```python
from build123d import *

# Parameters (mm, degrees)
SKETCH1_W           = 5
SKETCH1_H           = 15
BOSS_EXTRUDE1_DEPTH = 7
CUT_EXTRUDE3_REACH  = 90.347
SKETCH3_R           = 1.6
SKETCH3_4_R         = 2.2
CUT_EXTRUDE4_DEPTH  = 4
SKETCH4_R           = 2.2
CUT_EXTRUDE5_DEPTH  = 4


with BuildPart() as part:
    # Sketch1 → Boss-Extrude1 (new body)
    with BuildSketch(Plane(origin=(0, 0, 0), x_dir=(1, 0, 0), z_dir=(0, 1, 0))):
        Polygon((-68.342017383, -9.5), (-68.342017383, -49.5), (68.342017383, -49.5), (68.342017383, -9.5), (72.842017383, -9.5), (72.842017383, 9.5), (68.342017383, 9.5), (68.342017383, 49.5), (-68.342017383, 49.5), (-68.342017383, 9.5), (-72.842017383, 9.5), (-72.842017383, -9.5), align=None)
        with Locations((68.342017383, 0)):
            Rectangle(SKETCH1_W, SKETCH1_H, mode=Mode.SUBTRACT)
        with Locations((-68.342017383, 0)):
            Rectangle(SKETCH1_W, SKETCH1_H, mode=Mode.SUBTRACT)
    extrude(amount=BOSS_EXTRUDE1_DEPTH)

    # Sketch3 → Cut-Extrude3 (cut, up to next)
    with BuildSketch(Plane(origin=(0, 0, 0), x_dir=(1, 0, 0), z_dir=(0, 1, 0)), mode=Mode.PRIVATE) as cut_extrude3_sk1:
        with Locations(Location((-64.842017383, 46, 0), (0, 0, 270))):
            Circle(SKETCH3_R)
    cut_extrude3_tool1 = extrude(cut_extrude3_sk1.sketch, amount=CUT_EXTRUDE3_REACH, mode=Mode.PRIVATE) & part.part
    # Sketch3 → Cut-Extrude3 (cut, up to next)
    with BuildSketch(Plane(origin=(0, 0, 0), x_dir=(1, 0, 0), z_dir=(0, 1, 0)), mode=Mode.PRIVATE) as cut_extrude3_sk2:
        with Locations(Location((-64.842017383, -46, 0), (0, 0, 270))):
            Circle(SKETCH3_R)
    cut_extrude3_tool2 = extrude(cut_extrude3_sk2.sketch, amount=CUT_EXTRUDE3_REACH, mode=Mode.PRIVATE) & part.part
    # Sketch3 → Cut-Extrude3 (cut, up to next)
    with BuildSketch(Plane(origin=(0, 0, 0), x_dir=(1, 0, 0), z_dir=(0, 1, 0)), mode=Mode.PRIVATE) as cut_extrude3_sk3:
        with Locations(Location((64.842017383, -46, 0), (0, 0, 270))):
            Circle(SKETCH3_R)
    cut_extrude3_tool3 = extrude(cut_extrude3_sk3.sketch, amount=CUT_EXTRUDE3_REACH, mode=Mode.PRIVATE) & part.part
    # Sketch3 → Cut-Extrude3 (cut, up to next)
    with BuildSketch(Plane(origin=(0, 0, 0), x_dir=(1, 0, 0), z_dir=(0, 1, 0)), mode=Mode.PRIVATE) as cut_extrude3_sk4:
        with Locations(Location((64.842017383, 46, 0), (0, 0, 270))):
            Circle(SKETCH3_R)
    cut_extrude3_tool4 = extrude(cut_extrude3_sk4.sketch, amount=CUT_EXTRUDE3_REACH, mode=Mode.PRIVATE) & part.part
    add(cut_extrude3_tool1.solids().sort_by_distance((-64.842017, 0, -46))[0], mode=Mode.SUBTRACT)
    add(cut_extrude3_tool2.solids().sort_by_distance((-64.842017, 0, 46))[0], mode=Mode.SUBTRACT)
    add(cut_extrude3_tool3.solids().sort_by_distance((64.842017, 0, 46))[0], mode=Mode.SUBTRACT)
    add(cut_extrude3_tool4.solids().sort_by_distance((64.842017, 0, -46))[0], mode=Mode.SUBTRACT)

    # Sketch3_4 → Cut-Extrude4 (cut)
    with BuildSketch(Plane(origin=(0, 0, 0), x_dir=(1, 0, 0), z_dir=(0, 1, 0))):
        with Locations(Location((-37.5, 37.5, 0), (0, 0, 270))):
            Circle(SKETCH3_4_R)
        with Locations(Location((37.5, 37.5, 0), (0, 0, 270))):
            Circle(SKETCH3_4_R)
        with Locations(Location((37.5, -37.5, 0), (0, 0, 270))):
            Circle(SKETCH3_4_R)
        with Locations(Location((-37.5, -37.5, 0), (0, 0, 270))):
            Circle(SKETCH3_4_R)
    extrude(amount=CUT_EXTRUDE4_DEPTH, mode=Mode.SUBTRACT)

    # Sketch4 → Cut-Extrude5 (cut)
    with BuildSketch(Plane.XY.offset(49.5)):
        with Locations((0, 3.5)):
            Circle(SKETCH4_R)
        with Locations((10, 3.5)):
            Circle(SKETCH4_R)
        with Locations(Location((-10, 3.5, 0), (0, 0, 180))):
            Circle(SKETCH4_R)
    extrude(amount=-CUT_EXTRUDE5_DEPTH, mode=Mode.SUBTRACT)


solid = part.part
```
Design review of the part built by this model. Coordinates are the model's own, in mm. A direction names the side the tool comes from. Coordinates: 2 decimals unless noted, no trailing zeros. Order: outer loops, then holes, each group sorted by start corner. A loop starts at its lowest first (then second) coordinate and runs counter-clockwise, first axis right, second up. Notation, with made-up numbers: M 87.5,-20.5 L 126.5,-20.5 A13 ccw 126.5,-15.5 Z; hole C 71,-39.5 d7. An arc over 180 degrees is marked long. Answer as a JSON object with one key per item and string values. Group by question number.
1) For pin 1 (2 mm diameter, centred on y = 3, z = -26.5, fed in from +X); pin 2 (2.5 mm diameter, centred on x = 64.84, z = -46, fed in from +Y); pin 3 (1.3 mm diameter, centred on x = 38, z = 36.5, fed in from -Y); pin 4 (3 mm diameter, centred on y = 4.5, z = 17.5, fed in from -X), all flat-tipped, find the tip position at first contact; note any pin that passes through.
2) Wall thickness on L1, parallel to X at y = 3.25, z = 46; L2, parallel to Y at x = 0, z = 48; L3, parallel to X at y = 2.45, z = 37.5: over which ranges is each line inside the solid? List them lowest first.
3) Add section D-D, the plane x = -37.5. Write out the cut boundary in (y, z), then the cut area to 3 significant figures.
4) Tool access review of faces 1 (the flat face through (71, 3, 9.5)), 2 (the flat face through (10, 4, 45.5)), 3 (the flat face through (-65.842, 3, 0)): name each direction out of +Z, -Z, +X, -X, +Y, -Y from which nothing blocks a thin tool from reaching the whole face with its end or side.
5) Add section C-C, the plane x = -10. Write out the cut boundary in (y, z).
6) Add section A-A, the plane z = 1.5. Write out the cut boundary in (x, y), then the cut area to 3 significant figures.
7) Add section B-B, the plane z = -37.5. Write out the cut boundary in (x, y), then the cut area to 3 significant figures.
8) Mouldability with a two-part tool opening along Y and no side actions: class faces 4 (the flat face through (0, 4, 45.5)), 5 (the flat face through (-71, 3, -9.5)), 6 (the flat face through (-1, 7, -1)) as pulls with the +Y half, pulls with the -Y half, needs draft (parallel to the pull), parting line crosses it, or undercut.
Computed values:
{
 "1": {"pin 1": "stops at x = 68.34", "pin 2": "passes through", "pin 3": "stops at y = 4", "pin 4": "stops at x = -68.34"},
 "2": {"L1": "x = -68.34 to -66.44, -63.24 to -12.19, -7.81 to -2.19, 2.19 to 7.81, 12.19 to 63.24, 66.44 to 68.34", "L2": "y = 0 to 1.3, 5.7 to 7", "L3": "x = -68.34 to -39.7, -35.3 to 35.3, 39.7 to 68.34"},
 "3": {"outline": "M 0,-49.5 L 7,-49.5 L 7,49.5 L 0,49.5 L 0,39.7 L 4,39.7 L 4,35.3 L 0,35.3 L 0,-35.3 L 4,-35.3 L 4,-39.7 L 0,-39.7 Z", "area": "658 mm^2"},
 "4": {"face 1": "+Z, +X, +Y, -Y", "face 2": "+Z", "face 3": "+Y, -Y"},
 "5": {"outline": "M 0,-49.5 L 7,-49.5 L 7,49.5 L 5.7,49.5 L 5.7,45.5 L 1.3,45.5 L 1.3,49.5 L 0,49.5 Z"},
 "6": {"outline": "M -72.84,0 L -70.84,0 L -70.84,7 L -72.84,7 Z; M -65.84,0 L 65.84,0 L 65.84,7 L -65.84,7 Z; M 70.84,0 L 72.84,0 L 72.84,7 L 70.84,7 Z", "area": "950 mm^2"},
 "7": {"outline": "M -68.34,0 L -39.7,0 L -39.7,4 L -35.3,4 L -35.3,0 L 35.3,0 L 35.3,4 L 39.7,4 L 39.7,0 L 68.34,0 L 68.34,7 L -68.34,7 Z", "area": "922 mm^2"},
 "8": {"face 4": "undercut", "face 5": "needs draft", "face 6": "pulls with the +Y half"}
}
